Design review of the part shown in the three views and the two pictorial views. Dimensions are in mm from the part's minimum x, y and z. Round coordinates to 2 decimals unless told otherwise and drop trailing zeros. Write each loop counter-clockwise with the first axis right and the second up, starting at its lowest first coordinate (ties: lowest second). Pieces come first, ordered by that corner, then holes. Notation, with made-up numbers: (65.25, 77.5) - (97.25, 77.5) arc R20 ccw to (97.25, 105.5) - close; hole circle Ø5 at (38, -31). An arc over 180 degrees is marked (long way). Use one line per item in the form item = value.
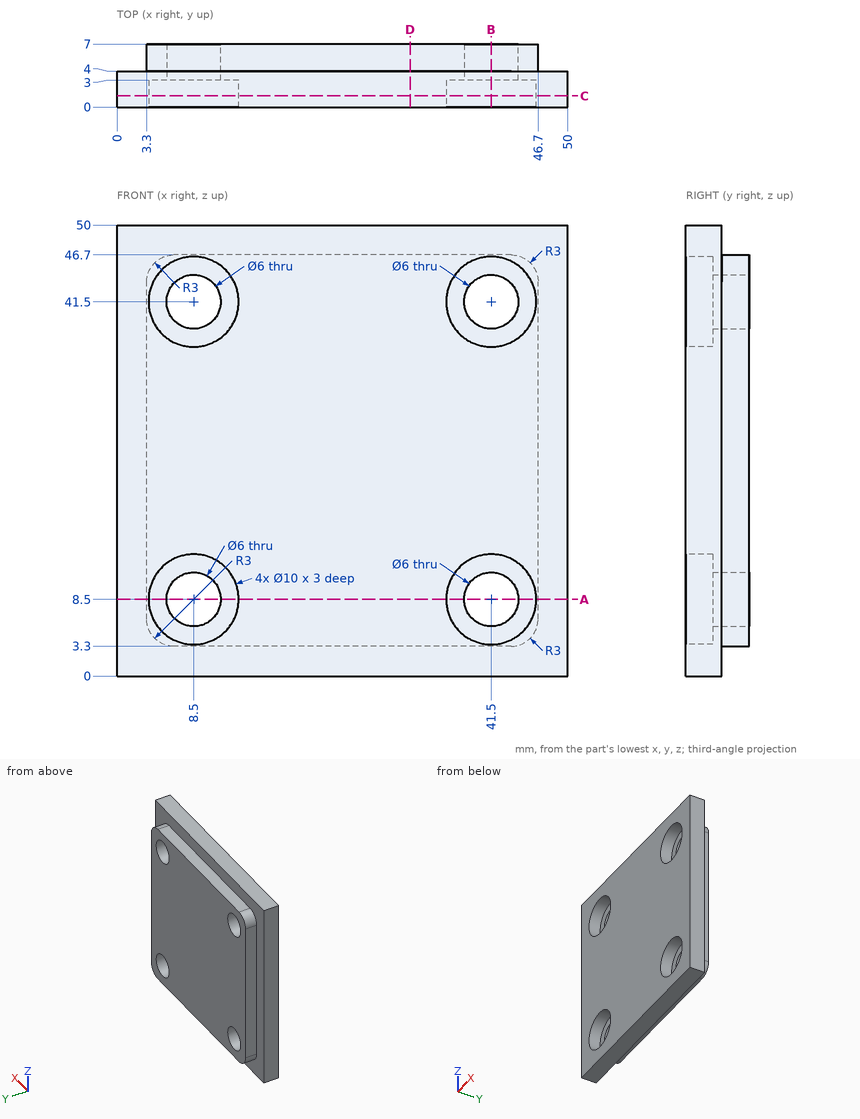
Q1. We need section C-C on y = 1.25. Write out the cut boundary in (x, z), then the cut area to 3 significant figures.
Calculated:
outline = (0, 0) - (50, 0) - (50, 50) - (0, 50) - close; hole circle Ø10 at (8.5, 8.5); hole circle Ø10 at (8.5, 41.5); hole circle Ø10 at (41.5, 8.5); hole circle Ø10 at (41.5, 41.5)
area = 2,190 mm2
Q2. We need section A-A on z = 8.5. Write out the cut boundary in (x, y), then the cut area to 3 significant figures.
Calculated:
outline = (0, 0) - (3.5, 0) - (3.5, 3) - (5.5, 3) - (5.5, 7) - (3.3, 7) - (3.3, 4) - (0, 4) - close; (11.5, 3) - (13.5, 3) - (13.5, 0) - (36.5, 0) - (36.5, 3) - (38.5, 3) - (38.5, 7) - (11.5, 7) - close; (44.5, 3) - (46.5, 3) - (46.5, 0) - (50, 0) - (50, 4) - (46.7, 4) - (46.7, 7) - (44.5, 7) - close
area = 222 mm2
Q3. We need section D-D on x = 32.5. Write out the cut boundary in (y, z).
Calculated:
outline = (0, 0) - (4, 0) - (4, 3.3) - (7, 3.3) - (7, 46.7) - (4, 46.7) - (4, 50) - (0, 50) - close
Q4. For P1, Ø7, axis at x = 8.5, z = 8.5, coming from the -Y side; P2, Ø0.9, axis at x = 18.5, y = 5.5, coming from the +Z side; P3, Ø2.5, axis at y = 5.5, z = 20, coming from the +X side, all flat-tipped, find the tip position at first contact; note any pin that passes through.
Calculated:
P1 = 3
P2 = 46.7
P3 = 46.7
Q5. To check wall thickness, follow line 1 along Z through (x, y) = (41.5, 4.25); line 2 along Z through (x, y) = (8.5, 1); line 3 along Z through (x, y) = (14, 5.25). State the ranges of each line that lie inside material, in increasing order. Write a range as from..to.
Calculated:
line_1 = 3.3..5.5, 11.5..38.5, 44.5..46.7
line_2 = 0..3.5, 13.5..36.5, 46.5..50
line_3 = 3.3..46.7
Q6. We need section B-B on x = 41.5. Write out the cut boundary in (y, z).
Calculated:
outline = (0, 0) - (4, 0) - (4, 3.3) - (7, 3.3) - (7, 5.5) - (3, 5.5) - (3, 3.5) - (0, 3.5) - close; (0, 13.5) - (3, 13.5) - (3, 11.5) - (7, 11.5) - (7, 38.5) - (3, 38.5) - (3, 36.5) - (0, 36.5) - close; (0, 46.5) - (3, 46.5) - (3, 44.5) - (7, 44.5) - (7, 46.7) - (4, 46.7) - (4, 50) - (0, 50) - close
